from build123d import *

# Parameters (mm, degrees)
F3_R = 25.4


with BuildPart() as f2:
    # F2: sweep along a path in F1
    with BuildLine(Plane.XY) as f2_path:
        Line((0, 0), (0, 101.6))
        Line((0, 101.6), (304.8, 101.6))
        Line((304.8, 101.6), (304.8, 203.2))
    # F0 (on Front) → F2 (sweep)
    with BuildSketch(Plane.XZ):
        Polygon((-19.05, 19.05), (-38.1, 19.05), (-38.1, -19.05), (38.1, -19.05), (38.1, 19.05), (19.05, 19.05), (19.05, 0), (-19.05, 0), align=None)
    sweep(path=f2_path.line, transition=Transition.RIGHT)

    # F3
    f3_edges = [f2.edges().sort_by_distance(p)[0] for p in [
        (342.9, 63.5, 0),
        (38.1, 63.5, 0),
        (-38.1, 139.7, 0),
        (266.7, 139.7, 0),
        (-19.05, 120.65, 9.525),
        (285.75, 120.65, 9.525),
        (19.05, 82.55, 9.525),
        (323.85, 82.55, 9.525),
    ]]
    fillet(f3_edges, radius=F3_R)


solid = f2.part
Verification items for the finished model (mm, model axes). A direction names the side the tool comes from. Coordinates: 2 decimals unless noted, no trailing zeros. Order: outer loops, then holes, each group sorted by start corner. A loop starts at its lowest first (then second) coordinate and runs counter-clockwise, first axis right, second up.
Item 1: Section check B-B, the plane y = 190.5. Enter the section's corners in (x, z), then the cut area to 3 significant figures.
Filled in:
outline: (266.7, -19.05) - (342.9, -19.05) - (342.9, 19.05) - (323.85, 19.05) - (323.85, 0) - (285.75, 0) - (285.75, 19.05) - (266.7, 19.05) - close
area: 2,180 mm2
Item 2: Section check C-C, the plane z = -9. Enter the section's corners in (x, y), then the cut area to 3 significant figures.
Filled in:
outline: (-38.1, 0) - (38.1, 0) - (38.1, 38.1) arc R25.4 cw to (63.5, 63.5) - (317.5, 63.5) arc R25.4 ccw to (342.9, 88.9) - (342.9, 203.2) - (266.7, 203.2) - (266.7, 165.1) arc R25.4 cw to (241.3, 139.7) - (-12.7, 139.7) arc R25.4 ccw to (-38.1, 114.3) - close
area: 38,700 mm2
Item 3: Depth check by flat-ended pin: pin 1 (8 mm diameter, centred on x = 197, z = -8, fed in from +Y); pin 2 (15 mm diameter, centred on y = 32, z = 11.5, fed in from +X); pin 3 (21 mm diameter, centred on x = 113, z = 7, fed in from -Y). Enter the tip coordinate at first touch or a pass-through.
Filled in:
pin 1: stops at y = 139.7
pin 2: stops at x = 38.14
pin 3: stops at y = 63.5
Item 4: Section check A-A, the plane z = 9.5. Enter the section's corners in (x, y).
Filled in:
outline: (-38.1, 0) - (-19.05, 0) - (-19.05, 95.25) arc R25.4 cw to (6.35, 120.65) - (260.35, 120.65) arc R25.4 ccw to (285.75, 146.05) - (285.75, 203.2) - (266.7, 203.2) - (266.7, 165.1) arc R25.4 cw to (241.3, 139.7) - (-12.7, 139.7) arc R25.4 ccw to (-38.1, 114.3) - close; (19.05, 0) - (38.1, 0) - (38.1, 38.1) arc R25.4 cw to (63.5, 63.5) - (317.5, 63.5) arc R25.4 ccw to (342.9, 88.9) - (342.9, 203.2) - (323.85, 203.2) - (323.85, 107.95) arc R25.4 cw to (298.45, 82.55) - (44.45, 82.55) arc R25.4 ccw to (19.05, 57.15) - close
Item 5: Material ranges on L1, parallel to X at y = 185.5, z = 12.5; L2, parallel to Y at x = 242, z = 6; L3, parallel to X at y = 183.5, z = -11.5, recorded low to high.
Filled in:
L1: x = 266.7 to 285.75, 323.85 to 342.9
L2: y = 63.5 to 82.55, 120.65 to 139.71
L3: x = 266.7 to 342.9
Item 6: Release check for a two-part mould opening along Y. For faces 6 (the face through (-11.81, 113.01, 9.39)), 7 (the face through (259.06, 146.94, 0.27)), 8 (the face through (135, 120.65, 9)) record: +Y half, -Y half, draft (parallel to the pull), parting line (faces both ways), or undercut.
Filled in:
face 6: -Y half
face 7: +Y half
face 8: undercut
Item 7: Section check D-D, the plane x = 103. Enter the section's corners in (y, z), then the cut area to 3 significant figures.
Filled in:
outline: (63.5, -19.05) - (139.7, -19.05) - (139.7, 19.05) - (120.65, 19.05) - (120.65, 0) - (82.55, 0) - (82.55, 19.05) - (63.5, 19.05) - close
area: 2,180 mm2
Item 8: Access from +Z, -Z, +X, -X, +Y, -Y to the whole of each face (thin tool, end or side, straight path). Record for faces 1 (the face through (173, 82.55, 10)), 2 (the face through (192, 63.5, 0)), 3 (the face through (285.75, 175, 9)), 4 (the face through (116, 139.7, 0)), 5 (the face through (19.05, 29, 10)).
Filled in:
face 1: +Z
face 2: +Z, -Z, +X, -Y
face 3: +Z, +Y
face 4: +Z, -Z, -X, +Y
face 5: +Z, -Y
